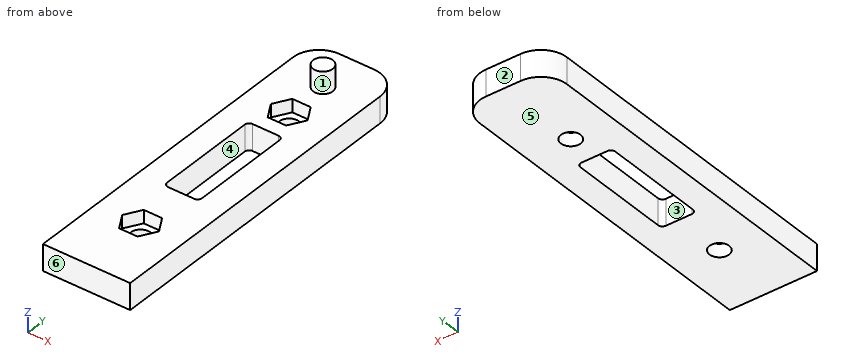
```python
from build123d import *

# Parameters (mm, degrees)
SKETCH_W        = 20
SKETCH_H        = 80
PAD_DEPTH       = 6
SKETCH001_R     = 2.25
PAD001_DEPTH    = 5
FILLET_R        = 6
SKETCH002_R     = 2.25
POCKET_DEPTH    = 8
POCKET001_DEPTH = 3
SKETCH004_W     = 8
SKETCH004_H     = 25
POCKET002_DEPTH = 7
FILLET001_R     = 1


with BuildPart() as part:
    # Sketch → Pad (new body)
    with BuildSketch(Plane.XY):
        with Locations((0, 40)):
            Rectangle(SKETCH_W, SKETCH_H)
    extrude(amount=PAD_DEPTH)

    # Sketch001 (on Face6 of Pad) → Pad001 (join)
    with BuildSketch(Plane.XY.offset(6)):
        with Locations((0, 70)):
            Circle(SKETCH001_R)
    extrude(amount=PAD001_DEPTH)

    # Fillet
    fillet_edges = [part.edges().sort_by_distance(p)[0] for p in [
        (-10, 80, 3),
        (10, 80, 3),
    ]]
    fillet(fillet_edges, radius=FILLET_R)

    # Sketch002 (on Face5 of Fillet) → Pocket (cut)
    with BuildSketch(Plane.XY.offset(6)):
        with Locations((0, 16)):
            Circle(SKETCH002_R)
        with Locations((0, 60)):
            Circle(SKETCH002_R)
    extrude(amount=-POCKET_DEPTH, mode=Mode.SUBTRACT)

    # Sketch003 (on Face5 of Pocket) → Pocket001 (cut)
    with BuildSketch(Plane.XY.offset(6)):
        Polygon((2.107328, 19.65), (-2.107328, 19.65), (-4.214657, 16), (-2.107328, 12.35), (2.107328, 12.35), (4.214657, 16), align=None)
        Polygon((2.107328, 56.35), (4.214657, 60), (2.107328, 63.65), (-2.107328, 63.65), (-4.214657, 60), (-2.107328, 56.35), align=None)
    extrude(amount=-POCKET001_DEPTH, mode=Mode.SUBTRACT)

    # Sketch004 (on Face5 of Pocket001) → Pocket002 (cut)
    with BuildSketch(Plane.XY.offset(6)):
        with Locations((0, 40.5)):
            Rectangle(SKETCH004_W, SKETCH004_H)
    extrude(amount=-POCKET002_DEPTH, mode=Mode.SUBTRACT)

    # Fillet001
    fillet001_edges = [part.edges().sort_by_distance(p)[0] for p in [
        (4, 53, 3),
        (-4, 53, 3),
        (-4, 28, 3),
        (4, 28, 3),
    ]]
    fillet(fillet001_edges, radius=FILLET001_R)


solid = part.part
```
Part model, mm, in its own coordinate system. Face numbers are marked on the shaded views. A direction names the side the tool comes from. Coordinates: 2 decimals unless noted, no trailing zeros. Order: outer loops, then holes, each group sorted by start corner. A loop starts at its lowest first (then second) coordinate and runs counter-clockwise, first axis right, second up. Notation, with made-up numbers: (81, 17) - (108, 17) arc R23 ccw to (108, 27) - close; hole circle Ø2 at (11.5, 8.5). An arc over 180 degrees is marked (long way). Return JSON: item names as keys, results as strings. Group by question number.
Item 1: Cut at D-D (y = 8.5). List the corners of the cut face in (x, z), plus the area to 3 significant figures.
Item 2: Cut at B-B (z = 2.25). List the corners of the cut face in (x, y).
Item 3: Cut at A-A (x = 0). List the corners of the cut face in (y, z).
Item 4: Pull direction Y, two halves, no side cores. Call the marked faces 4, 5 and 6: pulls with the +Y half, pulls with the -Y half, needs draft (parallel to the pull), parting line crosses it, or undercut.
Item 5: Cut at C-C (y = 70). List the corners of the cut face in (x, z), plus the area to 4 significant figures.
Item 6: Drill centre lines: probe 1 along Y at (x, z) = (0, 1.4); probe 2 along Y at (x, z) = (-1.25, 4.5); probe 3 along Z at (x, y) = (7, 13). Where is each one in solid material? Low to high. Write a range as from..to.
Item 7: Which spindle directions (+Z, -Z, +X, -X, +Y, -Y) get a long thin tool onto all of the face, cutting with end or side? Do the marked faces 1, 2 and 3. Say none if no direction does.
Item 8: Pin check, flat tips, straight feed: pin 1 (10 mm diameter, centred on x = -3.5, y = 35, fed in from +Z); pin 2 (5 mm diameter, centred on y = 9, z = 9.5, fed in from +X); pin 3 (6 mm diameter, centred on x = 0.5, y = 16, fed in from +Z). Stop position of each tip, or through.
Check values:
{
 "1": {"outline": "(-10, 0) - (10, 0) - (10, 6) - (-10, 6) - close", "area": "120 mm2"},
 "2": {"outline": "(-10, 0) - (10, 0) - (10, 74) arc R6 ccw to (4, 80) - (-4, 80) arc R6 ccw to (-10, 74) - close; hole (-4, 29) arc R1 ccw to (-3, 28) - (3, 28) arc R1 ccw to (4, 29) - (4, 52) arc R1 ccw to (3, 53) - (-3, 53) arc R1 ccw to (-4, 52) - close; hole circle Ø4.5 at (0, 16); hole circle Ø4.5 at (0, 60)"},
 "3": {"outline": "(0, 0) - (13.75, 0) - (13.75, 3) - (12.35, 3) - (12.35, 6) - (0, 6) - close; (18.25, 0) - (28, 0) - (28, 6) - (19.65, 6) - (19.65, 3) - (18.25, 3) - close; (53, 0) - (57.75, 0) - (57.75, 3) - (56.35, 3) - (56.35, 6) - (53, 6) - close; (62.25, 0) - (80, 0) - (80, 6) - (72.25, 6) - (72.25, 11) - (67.75, 11) - (67.75, 6) - (63.65, 6) - (63.65, 3) - (62.25, 3) - close"},
 "4": {"face 4": "undercut", "face 5": "needs draft", "face 6": "pulls with the -Y half"},
 "5": {"outline": "(-10, 0) - (10, 0) - (10, 6) - (2.25, 6) - (2.25, 11) - (-2.25, 11) - (-2.25, 6) - (-10, 6) - close", "area": "142.5 mm2"},
 "6": {"probe 1": "y = 0..13.75, 18.25..28, 53..57.75, 62.25..80", "probe 2": "y = 0..12.35, 19.65..28, 53..56.35, 63.65..80", "probe 3": "z = 0..6"},
 "7": {"face 1": "+Z", "face 2": "+Z, -Z, +X, -X, +Y", "face 3": "+Z, -Z"},
 "8": {"pin 1": "stops at z = 6", "pin 2": "passes through", "pin 3": "stops at z = 3"}
}
